```python
from build123d import *

# Parameters (mm, degrees)
BOSS_EXTRUDE1_DEPTH = 6.35
SKETCH5_R           = 2.032
CUT_EXTRUDE4_DEPTH  = 6.858
SKETCH6_R           = 2.286
CUT_EXTRUDE5_DEPTH  = 6.858
SKETCH7_R           = 2.078963723
SKETCH7_R_2         = 2.032
CUT_EXTRUDE6_DEPTH  = 44.972372637


with BuildPart() as part:
    # Sketch1 → Boss-Extrude1 (new body)
    with BuildSketch(Plane.XY):
        with BuildLine():
            Line((-39.734260423, 17.097332163), (-39.734260423, 11.839639722))
            ThreePointArc((-39.734260423, 11.839639722), (-39.446147588, 10.832316092), (-38.668957645, 10.129688385))
            Line((-38.668957645, 10.129688385), (11.411717792, -14.463177564))
            ThreePointArc((11.411717792, -14.463177564), (12.365282789, -14.803018024), (13.371011309, -14.91829111))
            Line((13.371011309, -14.91829111), (20.221726652, -14.91829111))
            ThreePointArc((20.221726652, -14.91829111), (20.670739459, -14.732303916), (20.856726652, -14.28329111))
            Line((20.856726652, -14.28329111), (20.856726652, 15.827332163))
            ThreePointArc((20.856726652, 15.827332163), (20.298765071, 17.174370581), (18.951726652, 17.732332163))
            Line((18.951726652, 17.732332163), (-39.099260423, 17.732332163))
            ThreePointArc((-39.099260423, 17.732332163), (-39.548273229, 17.546344969), (-39.734260423, 17.097332163))
        make_face()
        with BuildLine():
            Line((13.858514745, -7.578979228), (13.858514745, 10.493332163))
            ThreePointArc((13.858514745, 10.493332163), (13.300553163, 11.840370581), (11.953514745, 12.398332163))
            Line((11.953514745, 12.398332163), (-26.863603786, 12.398332163))
            ThreePointArc((-26.863603786, 12.398332163), (-27.605842685, 11.808742766), (-27.199482675, 10.952351628))
            Line((-27.199482675, 10.952351628), (12.394676227, -8.490953274))
            ThreePointArc((12.394676227, -8.490953274), (13.379754015, -8.441319049), (13.858514745, -7.578979228))
        make_face(mode=Mode.SUBTRACT)
    extrude(amount=BOSS_EXTRUDE1_DEPTH)

    # Sketch5 → Cut-Extrude4 (cut)
    with BuildSketch(Plane(origin=(0, 17.732332163, 0), x_dir=(1, 0, 0), z_dir=(0, 1, 0))):
        with Locations(Location((-21.503766885, -3.175, 0), (0, 0, 180))):
            Circle(SKETCH5_R)
        with Locations((1.356233115, -3.175)):
            Circle(SKETCH5_R)
    extrude(amount=-CUT_EXTRUDE4_DEPTH, mode=Mode.SUBTRACT)

    # Sketch6 → Cut-Extrude5 (cut)
    with BuildSketch(Plane(origin=(0, 17.732332163, 0), x_dir=(1, 0, 0), z_dir=(0, 1, 0))):
        with Locations(Location((-10.073766885, -3.175, 0), (0, 0, 180))):
            Circle(SKETCH6_R)
    extrude(amount=-CUT_EXTRUDE5_DEPTH, mode=Mode.SUBTRACT)

    # Sketch7 → Cut-Extrude6 (cut, through all)
    with BuildSketch(Plane(origin=(0, 0, 0), x_dir=(-1, 0, 0), z_dir=(0, 0, -1))):
        with Locations((33.883843897, 13.433671695)):
            Circle(SKETCH7_R)
        with Locations((-15.98734669, 14.538238486)):
            Circle(SKETCH7_R_2)
        with Locations((-15.98734669, -11.419081089)):
            Circle(SKETCH7_R_2)
    extrude(amount=-CUT_EXTRUDE6_DEPTH, mode=Mode.SUBTRACT)


solid = part.part
```
Can you work these out from the model? Positions are in its coordinate system, mm. A direction names the side the tool comes from. Round coordinates to 2 decimals unless told otherwise and drop trailing zeros. Loops run counter-clockwise (first coordinate to the right, second up) from the corner with the lowest first, then second, coordinate; pieces in that order, holes last.
Item 1: Suppose I cut it at D-D, the plane x = 17. Write out the boundary of the cut face in (y, z).
Item 2: If we mould it in two halves opening along X, with no side actions, what happens to faces 1 (the flat face through (-13.979, -1.995, 3.131)), 2 (the cylindrical face through (-35.804, 12.637, 3.131)), 3 (the flat face through (-10, 2, 0))? For each: +X half, -X half, draft (parallel to the pull), parting line (faces both ways), or undercut.
Item 3: Which directions (+Z, -Z, +X, -X, +Y, -Y) give clear straight access to the entire face, cutting with the end or side of a thin tool? Please do faces 4 (the cylindrical face through (13.315, 11.825, 3.131)), 5 (the cylindrical face through (-12.254, 15.103, 3.862)), 6 (the cylindrical face through (-39.45, 10.84, 3.13)).
Item 4: Suppose I cut it at C-C, the plane x = -5. Write out the boundary of the cut face in (y, z).
Item 5: Will these pins go through, and if not, where does the flat tip stop? pin 1 Ø3.5 at (x, z) = (-10.07, 3.18) entering from +Y; pin 2 Ø3 at (x, z) = (-13.5, 3) entering from -Y; pin 3 Ø3 at (y, z) = (2.5, 2.5) entering from -X.
Item 6: Please list where these lines run through material, in increasing order: L1, parallel to Y at x = 15, z = 2.25; L2, parallel to X at y = 13, z = 1.5; L3, parallel to X at y = 6.5, z = 1.75.
Item 7: Suppose I cut it at B-B, the plane y = -4. Write out the boundary of the cut face in (x, z).
Item 8: Suppose I cut it at A-A, the plane z = 1.75. State how many separate pieces and enclosed holes the cut face has, then the cut area to 3 significant figures.
Reported:
1. outline: (-14.92, 0) - (-13.18, 0) - (-13.18, 6.35) - (-14.92, 6.35) - close; (-9.66, 0) - (12.78, 0) - (12.78, 6.35) - (-9.66, 6.35) - close; (16.3, 0) - (17.73, 0) - (17.73, 6.35) - (16.3, 6.35) - close
2. face 1: -X half
2. face 2: undercut
2. face 3: draft
3. face 4: +Z, -Z
3. face 5: +Y
3. face 6: +Z, -Z, -X, -Y
4. outline: (-6.4, 0) - (0.05, 0) - (0.05, 6.35) - (-6.4, 6.35) - close; (12.4, 0) - (17.73, 0) - (17.73, 6.35) - (12.4, 6.35) - close
5. pin 1: stops at y = 3.4
5. pin 2: stops at y = -2.97
5. pin 3: stops at x = -26.19
6. L1: y = -14.92 to -13.2, -9.64 to 12.76, 16.31 to 17.73
6. L2: x = -39.73 to -35.92, -31.85 to -22.65, -20.35 to -11.63, -8.52 to 0.21, 2.51 to 14.66, 17.32 to 20.86
6. L3: x = -31.28 to -18.13, 13.86 to 20.86
7. outline: (-9.9, 0) - (3.25, 0) - (3.25, 6.35) - (-9.9, 6.35) - close; (13.86, 0) - (20.86, 0) - (20.86, 6.35) - (13.86, 6.35) - close
8. separate pieces: 3
8. enclosed holes: 3
8. area: 749 mm2
